Input: part model. Units: mm. Frame: model coordinates. Face numbers are marked on the shaded views. A direction names the side the tool comes from. Give positions to 0.01 mm unless a question says otherwise; leave off trailing zeros. Loops run counter-clockwise (first coordinate to the right, second up) from the corner with the lowest first, then second, coordinate; pieces in that order, holes last. Notation, with made-up numbers: (-3.5, 34.5) - (14.5, 34.5) arc R26 cw to (14.5, 72.5) - close; hole circle Ø4 at (42, -31). An arc over 180 degrees is marked (long way). Answer as a JSON object with one key per item and string values.
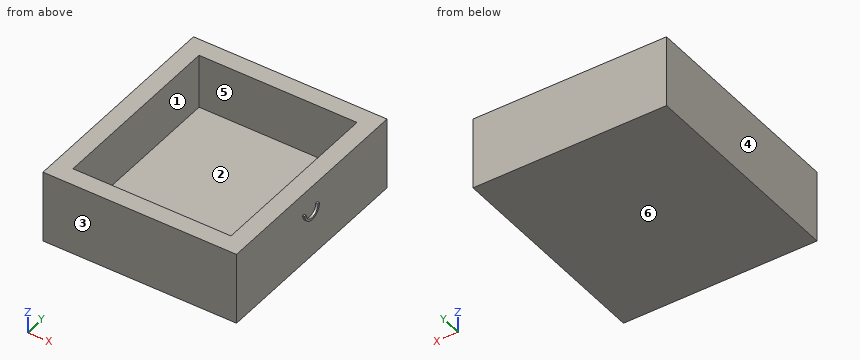
from build123d import *

# Parameters (mm, degrees)
F0_W     = 346
F0_H     = 129
F1_DEPTH = 195.7
F2_W     = 282.5
F2_H     = 327.9
F3_DEPTH = 97.25
F5_DEPTH = 4


# Not quite as in the source:
# - a feature names something its author has since deleted; it is built from what else it names


with BuildPart() as f1:
    # F0 (on Front) → F1 (new body, symmetric)
    with BuildSketch(Plane.XZ):
        Rectangle(F0_W, F0_H)
    extrude(amount=F1_DEPTH, both=True)

    # F2 (on face) → F3 (cut)
    with BuildSketch(Plane.XY.offset(64.5)):
        Rectangle(F2_W, F2_H)
    extrude(amount=-F3_DEPTH, mode=Mode.SUBTRACT)

    # F4 (on face) → F5 (join)
    with BuildSketch(Plane.YZ.offset(173)):
        with BuildLine():
            Line((-20.1823599637, 25.9178485721), (-23.953853175, 25.9178485721))
            ThreePointArc((-23.953853175, 25.9178485721), (-4.0838683271, 7.9147781718), (14.2255900428, 27.5027994066))
            Line((14.2255900428, 27.5027994066), (10.32506302, 27.5027994066))
            ThreePointArc((10.32506302, 27.5027994066), (-4.1526228185, 11.7732405564), (-20.1823599637, 25.9178485721))
        make_face()
    extrude(amount=F5_DEPTH)


solid = f1.part
Item 1: Cut plane B-B (x = -17). Return loops of the section in (y, z).
Geometry check:
{"outline": "(-195.7, -64.5) - (195.7, -64.5) - (195.7, 64.5) - (163.95, 64.5) - (163.95, -32.75) - (-163.95, -32.75) - (-163.95, 64.5) - (-195.7, 64.5) - close"}
Item 2: Cut plane C-C (y = 3). Return loops of the section in (x, z), then the cut area to 3 significant figures.
Geometry check:
{"outline": "(-173, -64.5) - (173, -64.5) - (173, 9.6) - (177, 9.6) - (177, 13.98) - (173, 13.98) - (173, 64.5) - (141.25, 64.5) - (141.25, -32.75) - (-141.25, -32.75) - (-141.25, 64.5) - (-173, 64.5) - close", "area": "17,200 mm2"}
Item 3: Cut plane A-A (y = -51). Return loops of the section in (x, z), then the cut area to 3 significant figures.
Geometry check:
{"outline": "(-173, -64.5) - (173, -64.5) - (173, 64.5) - (141.25, 64.5) - (141.25, -32.75) - (-141.25, -32.75) - (-141.25, 64.5) - (-173, 64.5) - close", "area": "17,200 mm2"}
Item 4: Material intervals for line 1 (Y direction, x = 1, z = 44); line 2 (X direction, y = -128.5, z = 43.5); line 3 (Z direction, x = -112.5, y = -99), sorted ascending. Write a range as [from, to].
Geometry check:
{"line 1": "y = [-195.7, -163.95], [163.95, 195.7]", "line 2": "x = [-173, -141.25], [141.25, 173]", "line 3": "z = [-64.5, -32.75]"}
Item 5: Mould query, pull axis Y, two halves, no side actions, for the marked faces 1, 2, 3 and 4. Classes: released by +Y, released by -Y, zero draft, split by the parting line, or undercut.
Geometry check:
{"face 1": "undercut", "face 2": "undercut", "face 3": "released by -Y", "face 4": "zero draft"}
Item 6: Contact query for flat-ended pins moving along their axis: P1, Ø3, axis at x = 175.5, y = 12.5, coming from the +Z side; P2, Ø8, axis at x = 74.5, y = 76.5, coming from the +Z side; P3, Ø2, axis at y = -21.5, z = 31, coming from the +X side. Output: stop coordinate, or through.
Geometry check:
{"P1": "stops at z = 27.5", "P2": "stops at z = -32.75", "P3": "stops at x = 173"}
Item 7: Access query for the marked faces 5 and 6. Directions: +Z, -Z, +X, -X, +Y, -Y. A direction counts if a zero-diameter tool reaches every point of the face in a straight line with its end or side. Return the directions, or none.
Geometry check:
{"face 5": "+Z", "face 6": "-Z, +X, -X, +Y, -Y"}
